Autodesk Inventor part; units mm, degrees
ref_plane "YZ Plane" through (0, 0, 0) normal (1, 0, 0) x (0, 1, 0)
ref_plane "XZ Plane" through (0, 0, 0) normal (0, 1, 0) x (-1, 0, 0)
ref_plane "XY Plane" through (0, 0, 0) normal (0, 0, 1) x (1, 0, 0)
sketch "Esboço1" plane through (0, 0, 0) normal (0, 1, 0) x (-1, 0, 0)
  line L0 (0, 0) -> (-91, 0)
  line L1 (-91, 0) -> (-91, -111)
  line L2 (-91, -111) -> (0, -111)
  line L3 (0, -111) -> (0, 0)
  line L4 (-3, -108) -> (-88, -108)
  line L5 (-88, -108) -> (-88, -3)
  line L6 (-88, -3) -> (-3, -3)
  line L7 (-3, -3) -> (-3, -108)
  dimension "d0" = 3
  dimension "d1" = 3
  dimension "d2" = 3
  dimension "d3" = 3
  dimension "d4" = 85
  dimension "d5" = 105
extrude "Extrusão1" add sketch "Esboço1" along normal blind 3 contours L4 L5 L6 L7
extrude "Extrusão2" add sketch "Esboço1" along normal blind 25
sketch "Esboço2" plane through (0, 0, 0) normal (0, 0, 1) x (1, 0, 0)
  circle A0 centre (20, 12) radius 3
  circle A1 centre (66, 13) radius 3.75
  line L0 (0, 0) -> (0, 25)
  line L1 (91, 0) -> (91, 25)
  circle A2 centre (35, 12) radius 3
  line L2 (0, 0) -> (91, 0)
  point P0 (0, 12.5)
  dimension "d10" = 6
  dimension "d11" = 7.5
  dimension "d25" = 20
  dimension "d26" = 25
  dimension "d27" = 6
  dimension "d28" = 15
  dimension "d29" = 12
  dimension "d30" = 13
  dimension "d31" = 12
extrude "Extrusão3" cut sketch "Esboço2" against normal blind 30
sketch "Esboço3" plane through (91, 0, 0) normal (1, 0, 0) x (0, 0, -1)
  circle A0 centre (16.1671, 10) radius 1.5
  circle A1 centre (34.0898, 10) radius 1.5
  circle A2 centre (25.3707, 10) radius 1.5
  line L0 (0, 0) -> (111, 0)
  dimension "d14" = 3
  dimension "d15" = 3
  dimension "d16" = 3
  dimension "d32" = 10
  dimension "d33" = 10
  dimension "d34" = 10
extrude "Extrusão4" cut sketch "Esboço3" against normal blind 10
sketch "Esboço4" plane through (0, 3, 0) normal (0, 1, 0) x (1, 0, 0)
  line L0 (28.1, 81.6) -> (63, 81.6)
  line L1 (63, 81.6) -> (63, 98)
  line L2 (63, 98) -> (28.1, 98)
  line L3 (28.1, 98) -> (28.1, 81.6)
  line L4 (88, 108) -> (88, 3)
  line L5 (3, 108) -> (88, 108)
  point P0 (0, 0)
  point P1 (63, 89.8)
  dimension "d19" = 34.9
  dimension "d20" = 16.4
  dimension "d23" = 25
  dimension "d24" = 10
extrude "Extrusão5" cut sketch "Esboço4" against normal blind 1.5
properties part number "Caixa_3DPrint"
Input: part model. Units: mm. Frame: model coordinates. A direction names the side the tool comes from. Round coordinates to 2 decimals unless told otherwise and drop trailing zeros. Write each loop counter-clockwise with the first axis right and the second up, starting at its lowest first coordinate (ties: lowest second). Pieces come first, ordered by that corner, then holes.
1) Reachability of faces 1 (the flat face through (91, 12, -55)), 2 (the cylindrical face through (17, 12, -1)), 3 (the flat face through (45, 1.5, -90)), 4 (the cylindrical face through (89.52, 10.45, -17.6)) from +Z, -Z, +X, -X, +Y, -Y: full face, straight path, thin tool, end or side. Return the list, or none.
2) Ray query, L1, parallel to Z at x = 12.5, y = 21.5; L2, parallel to X at y = 3.75, z = -47; L3, parallel to Y at x = 20, z = -1.85. Return the intervals inside material, ascending.
3) Cut plane C-C (x = 47.5). Return the cut outline in (y, z), then the cut area to 3 significant figures.
4) Cut plane B-B (y = 23.5). Return the cut outline in (x, z).
5) Draft query along Z for faces 5 (the flat face through (46, 12, -111)), 6 (the flat face through (90, 25, -55)), 7 (the flat face through (46, 14, -3)). Return one class per face: pulls with the +Z half, pulls with the -Z half, needs draft (parallel to the pull), parting line crosses it, or undercut.
6) Cut plane A-A (x = 35). Return the cut outline in (y, z), then the cut area to 3 significant figures.
7) Contact query for flat-ended pins moving along their axis: P1, Ø13, axis at x = 52, z = -88, coming from the +Y side; P2, Ø7, axis at x = 66, y = 13, coming from the +Z side. Output: stop coordinate, or through.
8) Cut plane D-D (z = -52). Return the cut outline in (x, y), then the cut area to 3 significant figures.
Geometry says:
1. face 1: +Z, -Z, +X, +Y, -Y
1. face 2: +Z
1. face 3: +Y
1. face 4: +X
2. L1: z = -111 to -108, -3 to 0
2. L2: x = 0 to 3, 88 to 91
2. L3: y = 0 to 9, 15 to 25
3. outline: (0, -111) - (25, -111) - (25, -108) - (3, -108) - (3, -98) - (1.5, -98) - (1.5, -81.6) - (3, -81.6) - (3, -3) - (25, -3) - (25, 0) - (0, 0) - close
3. area: 440 mm2
4. outline: (0, -111) - (91, -111) - (91, 0) - (0, 0) - close; hole (3, -108) - (88, -108) - (88, -3) - (3, -3) - close
5. face 5: pulls with the -Z half
5. face 6: needs draft
5. face 7: undercut
6. outline: (0, -111) - (25, -111) - (25, -108) - (3, -108) - (3, -98) - (1.5, -98) - (1.5, -81.6) - (3, -81.6) - (3, -3) - (9, -3) - (9, 0) - (0, 0) - close; (15, -3) - (25, -3) - (25, 0) - (15, 0) - close
6. area: 422 mm2
7. P1: stops at y = 3
7. P2: stops at z = -108
8. outline: (0, 0) - (91, 0) - (91, 25) - (88, 25) - (88, 3) - (3, 3) - (3, 25) - (0, 25) - close
8. area: 405 mm2
